The listing builds one solid part. Answer for the finished solid, in the listing's coordinates (mm). A direction names the side the tool comes from. Round coordinates to 2 decimals unless told otherwise and drop trailing zeros. Write each loop counter-clockwise with the first axis right and the second up, starting at its lowest first coordinate (ties: lowest second). Pieces come first, ordered by that corner, then holes. Notation, with made-up numbers: M 30,70.5 L 34,70.5 A31 ccw 34,102.5 Z; hole C 48.25,3 d3. An arc over 180 degrees is marked long. Put each result on its own line as item: value. Start each with the question number.
```python
from build123d import *

# Parameters (mm, degrees)
F1_DEPTH  = 9
F3_DEPTH  = 6.5
F5_DEPTH  = 5
F7_DEPTH  = 5
F9_DEPTH  = 11.3
F11_DEPTH = 3
F13_DEPTH = 2
F15_DEPTH = 2


with BuildPart() as f1:
    # F0 (on Front) → F1 (new body)
    with BuildSketch(Plane.XZ):
        with BuildLine():
            Line((31.35, 71), (-31.35, 71))
            ThreePointArc((-31.35, 71), (-34.8855339059, 69.5355339059), (-36.35, 66))
            Line((-36.35, 66), (-36.35, -66))
            ThreePointArc((-36.35, -66), (-34.8855339059, -69.5355339059), (-31.35, -71))
            Line((-31.35, -71), (31.35, -71))
            ThreePointArc((31.35, -71), (34.8855339059, -69.5355339059), (36.35, -66))
            Line((36.35, -66), (36.35, 66))
            ThreePointArc((36.35, 66), (34.8855339059, 69.5355339059), (31.35, 71))
        make_face()
    extrude(amount=F1_DEPTH)

    # F2 (on face) → F3 (cut)
    with BuildSketch(Plane.XZ.offset(9)):
        with BuildLine():
            Line((33, 69.25), (-33, 69.25))
            ThreePointArc((-33, 69.25), (-33.7071067812, 68.9571067812), (-34, 68.25))
            Line((-34, 68.25), (-34, -68.25))
            ThreePointArc((-34, -68.25), (-33.7071067812, -68.9571067812), (-33, -69.25))
            Line((-33, -69.25), (33, -69.25))
            ThreePointArc((33, -69.25), (33.7071067812, -68.9571067812), (34, -68.25))
            Line((34, -68.25), (34, 68.25))
            ThreePointArc((34, 68.25), (33.7071067812, 68.9571067812), (33, 69.25))
        make_face()
    extrude(amount=-F3_DEPTH, mode=Mode.SUBTRACT)

    # F4 (on face) → F5 (cut)
    with BuildSketch(Plane.YZ.offset(36.35)):
        with BuildLine():
            Line((-4.6452410497, 26.2636251819), (-2.8310960583, 26.2636251819))
            Line((-2.8310960583, 26.2636251819), (0, 26.2636251819))
            Line((0, 26.2636251819), (0, 44.2636251819))
            Line((0, 44.2636251819), (-1.15, 44.2636251819))
            Line((-1.15, 44.2636251819), (-6.238168554, 44.2636251819))
            Line((-6.238168554, 44.2636251819), (-6.326337108, 44.2636251819))
            Line((-6.326337108, 44.2636251819), (-7.738168554, 44.2636251819))
            ThreePointArc((-7.738168554, 44.2636251819), (-8.4452753352, 43.9707319631), (-8.738168554, 43.2636251819))
            Line((-8.738168554, 43.2636251819), (-8.738168554, 27.2636251819))
            ThreePointArc((-8.738168554, 27.2636251819), (-8.4452753352, 26.5565184007), (-7.738168554, 26.2636251819))
            Line((-7.738168554, 26.2636251819), (-4.6452410497, 26.2636251819))
        make_face()
        with BuildLine():
            Line((0, 44.2636251819), (0, 26.2636251819))
            Line((0, 26.2636251819), (0.261831446, 26.2636251819))
            ThreePointArc((0.261831446, 26.2636251819), (0.9689382272, 26.5565184007), (1.261831446, 27.2636251819))
            Line((1.261831446, 27.2636251819), (1.261831446, 43.2636251819))
            ThreePointArc((1.261831446, 43.2636251819), (0.9689382272, 43.9707319631), (0.261831446, 44.2636251819))
            Line((0.261831446, 44.2636251819), (0, 44.2636251819))
        make_face()
    extrude(amount=-F5_DEPTH, mode=Mode.SUBTRACT)

    # F6 (on face) → F7 (cut)
    with BuildSketch(Plane(origin=(-36.35, 0, 0), x_dir=(0, -1, 0), z_dir=(-1, 0, 0))):
        Polygon((0, 53.926020956), (0, 11.926020956), (1.3606869444, 11.926020956), (5.3289291725, 11.926020956), (7.5948080584, 11.926020956), (8.6544789374, 11.9307097048), (8.6544789374, 53.926020956), (6.6106869444, 53.926020956), (5.3289291725, 53.926020956), (1.3606869444, 53.926020956), align=None)
        with BuildLine():
            ThreePointArc((-5.1551919416, 12.926020956), (-4.8622987227, 12.2189141749), (-4.1551919416, 11.926020956))
            Line((-4.1551919416, 11.926020956), (0, 11.926020956))
            Line((0, 11.926020956), (0, 53.926020956))
            Line((0, 53.926020956), (-4.2237708107, 53.926020956))
            ThreePointArc((-4.2237708107, 53.926020956), (-4.9107913061, 53.5846351538), (-5.1551919416, 52.8574420869))
            Line((-5.1551919416, 52.8574420869), (-5.1551919416, 12.926020956))
        make_face()
    extrude(amount=-F7_DEPTH, mode=Mode.SUBTRACT)

    # F8 (on face) → F9 (cut)
    with BuildSketch(Plane(origin=(0, 0, -71), x_dir=(1, 0, 0), z_dir=(0, 0, -1))):
        with BuildLine():
            Line((-23.15, 2.6055127643), (23.15, 2.6055127643))
            ThreePointArc((23.15, 2.6055127643), (23.8571067812, 2.8984059831), (24.15, 3.6055127643))
            Line((24.15, 3.6055127643), (24.15, 5.5759565953))
            Line((24.15, 5.5759565953), (-24.15, 5.6350689333))
            Line((-24.15, 5.6350689333), (-24.15, 3.6055127643))
            ThreePointArc((-24.15, 3.6055127643), (-23.8571067812, 2.8984059831), (-23.15, 2.6055127643))
        make_face()
        with BuildLine():
            Line((-24.15, 5.6350689333), (24.15, 5.5759565953))
            Line((24.15, 5.5759565953), (24.15, 7.6055127643))
            ThreePointArc((24.15, 7.6055127643), (23.8571067812, 8.3126195455), (23.15, 8.6055127643))
            Line((23.15, 8.6055127643), (-23.15, 8.6055127643))
            ThreePointArc((-23.15, 8.6055127643), (-23.8571067812, 8.3126195455), (-24.15, 7.6055127643))
            Line((-24.15, 7.6055127643), (-24.15, 5.6350689333))
        make_face()
    extrude(amount=-F9_DEPTH, mode=Mode.SUBTRACT)

    # F10 (on face) → F11 (cut)
    with BuildSketch(Plane(origin=(0, 0, 0), x_dir=(-1, 0, 0), z_dir=(0, 1, 0))):
        with BuildLine():
            ThreePointArc((-29.8940427601, 55.4671416283), (-29.6011495413, 54.7600348471), (-28.8940427601, 54.4671416283))
            Line((-28.8940427601, 54.4671416283), (1.1059572399, 54.4671416283))
            ThreePointArc((1.1059572399, 54.4671416283), (1.8130640211, 54.7600348471), (2.1059572399, 55.4671416283))
            Line((2.1059572399, 55.4671416283), (2.1059572399, 65.6569396853))
            ThreePointArc((2.1059572399, 65.6569396853), (1.8130640211, 66.3640464665), (1.1059572399, 66.6569396853))
            Line((1.1059572399, 66.6569396853), (-28.8940427601, 66.6569396853))
            ThreePointArc((-28.8940427601, 66.6569396853), (-29.6011495413, 66.3640464665), (-29.8940427601, 65.6569396853))
            Line((-29.8940427601, 65.6569396853), (-29.8940427601, 55.4671416283))
        make_face()
    extrude(amount=-F11_DEPTH, mode=Mode.SUBTRACT)

    # F12 (on face) → F13 (join)
    with BuildSketch(Plane.XZ.offset(9)):
        with BuildLine():
            Line((31.35, 71), (-31.35, 71))
            ThreePointArc((-31.35, 71), (-34.8855339059, 69.5355339059), (-36.35, 66))
            Line((-36.35, 66), (-36.35, -66))
            ThreePointArc((-36.35, -66), (-34.8855339059, -69.5355339059), (-31.35, -71))
            Line((-31.35, -71), (31.35, -71))
            ThreePointArc((31.35, -71), (34.8855339059, -69.5355339059), (36.35, -66))
            Line((36.35, -66), (36.35, 66))
            ThreePointArc((36.35, 66), (34.8855339059, 69.5355339059), (31.35, 71))
        make_face()
    extrude(amount=F13_DEPTH)

    # F14 (on face) → F15 (cut)
    with BuildSketch(Plane.XZ.offset(11)):
        with BuildLine():
            Line((27.5, 66), (-23.9265979081, 66))
            Line((-23.9265979081, 66), (-27.5, 66))
            ThreePointArc((-27.5, 66), (-31.0355339059, 64.5355339059), (-32.5, 61))
            Line((-32.5, 61), (-32.5, -61))
            ThreePointArc((-32.5, -61), (-31.0355339059, -64.5355339059), (-27.5, -66))
            Line((-27.5, -66), (27.5, -66))
            ThreePointArc((27.5, -66), (31.0355339059, -64.5355339059), (32.5, -61))
            Line((32.5, -61), (32.5, 61))
            ThreePointArc((32.5, 61), (31.0355339059, 64.5355339059), (27.5, 66))
        make_face()
    extrude(amount=-F15_DEPTH, mode=Mode.SUBTRACT)


solid = f1.part
```
Item 1: Section C-C (x = -6.5) is taken. Give the vertices of the cut face in (y, z), and give its area (3 significant figures).
Item 2: Which of the six approach directions +Z, -Z, +X, -X, +Y, -Y give full straight-line access (tool end or side, diameter ignored) to faces 5 (the flat face through (0, -6, 69.25)), 6 (the cylindrical face through (-31, -10.01, 64.57)), 7 (the flat face through (31.35, -1, 35)), 8 (the flat face through (34.4, -3.1, 26.264))?
Item 3: Section D-D (z = -46) is taken. Give the vertices of the cut face in (x, y), and give its area (3 significant figures).
Item 4: Section A-A (y = -6) is taken. Give the vertices of the cut face in (x, z).
Item 5: Flat-ended cylindrical pins translate along their axes: pin 1 (0.7 mm diameter, centred on x = -35, z = 41, fed in from +Y); pin 2 (3 mm diameter, centred on y = -1.5, z = 35.5, fed in from -X); pin 3 (1.5 mm diameter, centred on x = -35, y = -4, fed in from -Z). Find the tip coordinate at first contact, or state that the pin passes through.
Item 6: Consider line 1 along X through (y, z) = (-9.25, 4.5); line 2 along Z through (x, y) = (28, -8); line 3 along X through (y, z) = (-3.75, 62.5). Determine where each line is inside the solid, lowest interval first. Write a range as [from, to].
Item 7: Determine the mould class of faces 1 (the cylindrical face through (34.92, -5.42, 69.5)), 2 (the flat face through (-35, -11, 0)), 3 (the flat face through (34.4, -3, 44.264)), 4 (the cylindrical face through (-34.92, -5.42, -69.5)) for opening direction Z: released by +Z, released by -Z, zero draft, split by the parting line, or undercut.
Item 8: Section B-B (x = 6) is taken. Give the vertices of the cut face in (y, z), and give its area (3 significant figures).
Output values:
1. outline: M -11,-71 L -8.61,-71 L -8.61,-69.25 L -9,-69.25 L -9,-66 L -11,-66 Z; M -11,66 L -9,66 L -9,69.25 L -2.5,69.25 L -2.5,-69.25 L -2.61,-69.25 L -2.61,-71 L 0,-71 L 0,71 L -11,71 Z
1. area: 387 mm^2
2. face 5: none
2. face 6: -Y
2. face 7: +X, +Y, -Y
2. face 8: +X, +Y
3. outline: M -36.35,-11 L -32.5,-11 L -32.5,-9 L -34,-9 L -34,-2.5 L 34,-2.5 L 34,-9 L 32.5,-9 L 32.5,-11 L 36.35,-11 L 36.35,0 L -36.35,0 Z
3. area: 228 mm^2
4. outline: M -36.35,-66 A5 ccw -31.35,-71 L -24.15,-71 L -24.15,-69.25 L -33,-69.25 A1 cw -34,-68.25 L -34,11.93 L -36.35,11.93 Z; M -36.35,53.93 L -34,53.93 L -34,68.25 A1 cw -33,69.25 L 33,69.25 A1 cw 34,68.25 L 34,44.26 L 36.35,44.26 L 36.35,66 A5 ccw 31.35,71 L -31.35,71 A5 ccw -36.35,66 Z; M 24.15,-71 L 31.35,-71 A5 ccw 36.35,-66 L 36.35,26.26 L 34,26.26 L 34,-68.25 A1 cw 33,-69.25 L 24.15,-69.25 Z
5. pin 1: stops at y = -8.65
5. pin 2: stops at x = -31.35
5. pin 3: stops at z = -70.07
6. line 1: x = [-36.35, -32.5], [32.5, 36.35]
6. line 2: z = [-71, -69.25], [69.25, 71]
6. line 3: x = [-36.35, -34], [34, 36.35]
7. face 1: released by +Z
7. face 2: zero draft
7. face 3: undercut
7. face 4: released by -Z
8. outline: M -11,-71 L -8.61,-71 L -8.61,-69.25 L -9,-69.25 L -9,-66 L -11,-66 Z; M -11,66 L -9,66 L -9,69.25 L -2.5,69.25 L -2.5,66.66 L 0,66.66 L 0,71 L -11,71 Z; M -2.61,-71 L 0,-71 L 0,54.47 L -2.5,54.47 L -2.5,-69.25 L -2.61,-69.25 Z
8. area: 357 mm^2
